Check sheet for the drawn part. Datum: minimum x, y, z corner. Units: mm. A direction names the side the tool comes from. Coordinates: 2 decimals unless noted, no trailing zeros. Write each loop counter-clockwise with the first axis right and the second up, starting at its lowest first coordinate (ties: lowest second). Pieces come first, ordered by that corner, then holes. Notation, with made-up numbers: (35, -29) -> (76, -29) arc R21 ccw to (76, 3) -> close; hole circle Ø4 at (-15, -2.5). An arc over 180 degrees is marked (long way). Write item = value, one per line. Start each with the question number.
(1) Section check A-A (y = 5). Record the cut outline in (x, z) (3 decimals), plus the area to 3 significant figures.
(2) Gauge pin test, flat ends, axial feed: pin 1 Ø1.5 at (x, y) = (5, 5.5) entering from +Z; pin 2 Ø2 at (y, z) = (4.5, 27) entering from +X; pin 3 Ø2 at (y, z) = (6, 24) entering from +X; pin 4 Ø3 at (x, y) = (22.5, 2) entering from +Z. Record the tip position at first contact, or that the pin passes through.
(3) Section check C-C (z = 19.5). Record the cut outline in (x, y).
(4) Material ranges on probe 1 along X at (y, z) = (0.4, 28.5); probe 2 along Z at (x, y) = (47.5, 0.7); probe 3 along Y at (x, z) = (16, 21.5), recorded low to high. Write a range as [from, to].
(5) Section check B-B (x = 47.5). Record the cut outline in (y, z).
(6) Section check D-D (z = 24). Record the cut outline in (x, y), plus the area to 3 significant figures.
(7) Set-up check for the marked faces 1, 2 and 3: record each of +Z, -Z, +X, -X, +Y, -Y from which the full face is reachable in a straight line by a thin tool's end or side.
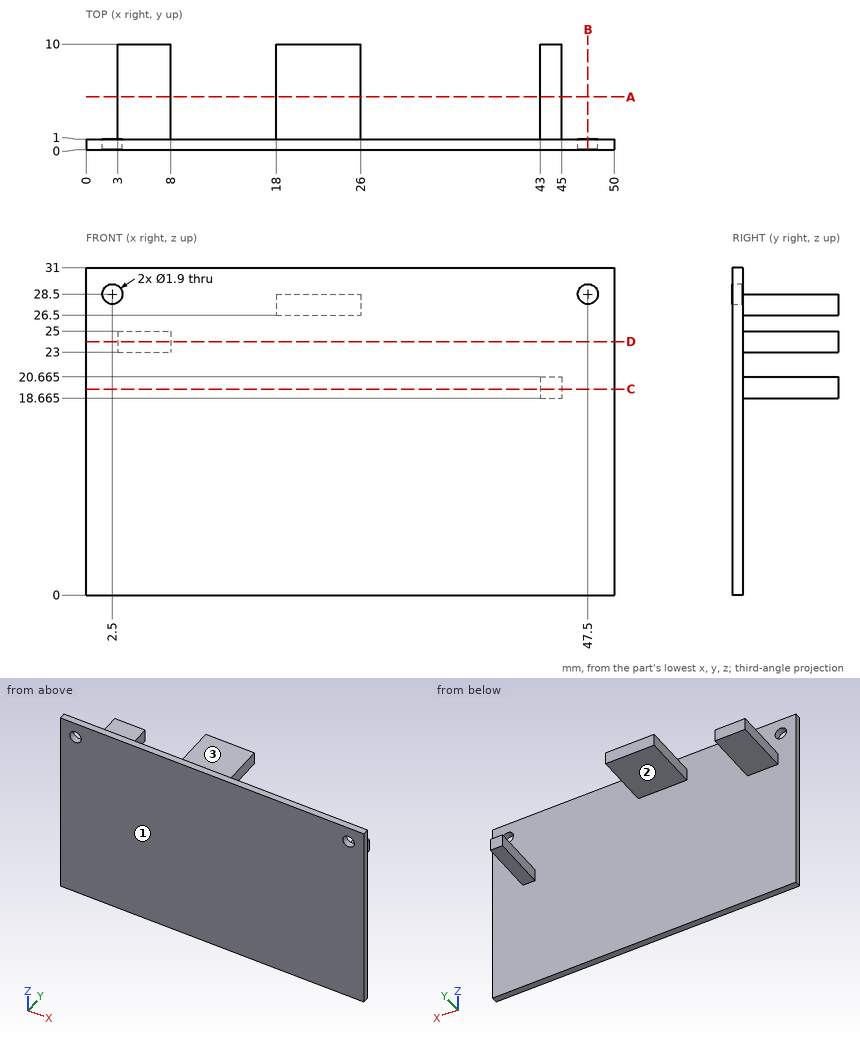
Response:
q1.outline = (3, 23) -> (8, 23) -> (8, 25) -> (3, 25) -> close; (18, 26.5) -> (26, 26.5) -> (26, 28.5) -> (18, 28.5) -> close; (43, 18.665) -> (45, 18.665) -> (45, 20.665) -> (43, 20.665) -> close
q1.area = 30.0 mm2
q2.pin_1 = 25
q2.pin_2 = 26
q2.pin_3 = 8
q2.pin_4 = 31
q3.outline = (0, 0) -> (50, 0) -> (50, 1) -> (45, 1) -> (45, 10) -> (43, 10) -> (43, 1) -> (0, 1) -> close
q4.probe_1 = [0, 1.55], [3.45, 46.55], [48.45, 50]
q4.probe_2 = [0, 27.55], [29.45, 31]
q4.probe_3 = [0, 1]
q5.outline = (0, 0) -> (1, 0) -> (1, 27.55) -> (0, 27.55) -> close; (0, 29.45) -> (1, 29.45) -> (1, 31) -> (0, 31) -> close
q6.outline = (0, 0) -> (50, 0) -> (50, 1) -> (8, 1) -> (8, 10) -> (3, 10) -> (3, 1) -> (0, 1) -> close
q6.area = 95.0 mm2
q7.face_1 = +Z, -Z, +X, -X, -Y
q7.face_2 = -Z, +X, -X, +Y
q7.face_3 = +Z, +X, -X, +Y
